Design review of the part built by this model. Coordinates are the model's own, in mm. A direction names the side the tool comes from. Coordinates: 2 decimals unless noted, no trailing zeros. Loops run counter-clockwise (first coordinate to the right, second up) from the corner with the lowest first, then second, coordinate; pieces in that order, holes last. Notation, with made-up numbers: M -6,86 L 27,86 A18 cw 27,91 Z; hole C 26.25,33.25 d7. An arc over 180 degrees is marked long. Answer as a JSON object with one key per item and string values. Group by question number.
1. Draft analysis for pull direction Z (two halves, no side actions). For faces 1 (the flat face through (10, 0, 0)), 2 (the flat face through (0, -10.922, 10)), 3 (the cylindrical face through (-0.123, 0.248, -12.303)), 4 (the flat face through (10, 0, 20.32)), state which applies: +Z half, -Z half, draft (parallel to the pull), parting line (faces both ways), or undercut.
2. Machinability: for faces 5 (the flat face through (-10, 0, 20.32)), 6 (the flat face through (8.763, -2, -7)), 7 (the flat face through (8.763, -2, 28)), which of the approach directions +Z, -Z, +X, -X, +Y, -Y give a long, thin tool a straight path to every point of the face, cutting with its end or side? Answer none if there is none.
3. Insertion check: pin 1 (3 mm diameter, centred on x = -5, z = -6, fed in from +Y); pin 2 (3 mm diameter, centred on x = 10, y = -3, fed in from -Z); pin 3 (3 mm diameter, centred on x = -10.5, y = 3, fed in from +Z); pin 4 (3 mm diameter, centred on y = 0, z = -10.414, fed in from -X). Each pin has a flat end and moves straight along its axis. Give the tip position at first contact, or say it passes through.
4. Consider section C-C (z = -2). State the section outline as (x, y) points.
5. Consider section A-A (y = 5.5). State the section outline as (x, z) points, then the cut area to 3 significant figures.
6. To check wall thickness, follow probe 1 along Z at (x, y) = (2.25, 0); probe 2 along X at (y, z) = (-6.35, -4.5); probe 3 along Y at (x, z) = (1.25, 1). State the ranges of each line that lie inside material, in increasing order.
7. Consider section D-D (x = 0). Count the separate pieces of the cut face and the enclosed holes in it, then the cut area to 3 significant figures.
8. Consider section B-B (x = -3.5). State the section outline as (y, z) points (3 decimals), then the cut area to 3 significant figures.
from build123d import *

# Parameters (mm, degrees)
SKETCH1_R               = 12.7
FINGERBODY_DEPTH        = 20.32
SKETCH2_W               = 17.526
SKETCH2_H               = 18.384757926
BOSS_EXTRUDE2_DEPTH     = 16.51
SKETCH4_R               = 1.905
CUT_EXTRUDE2_DEPTH      = 45.479200409
CUT_EXTRUDE3_DEPTH      = 45.479200409
FILLET2_R               = 2.54
CUT_EXTRUDE5_DEPTH      = 41.975955144
FILLET3_R               = 1.524
FILLET4_R               = 1.524
FILLET6_R               = 1.524
CUT_EXTRUDE6_DEPTH      = 41.460214887
CUT_EXTRUDE6_DEPTH_BACK = 41.460214887
SKETCH11_R              = 2.413


with BuildPart() as part:
    # Sketch1 → FingerBody (new body)
    with BuildSketch(Plane.XY):
        Circle(SKETCH1_R)
    extrude(amount=FINGERBODY_DEPTH)

    # Sketch2 → Boss-Extrude2 (add)
    with BuildSketch(Plane(origin=(0, 0, 0), x_dir=(-1, 0, 0), z_dir=(0, 0, -1))):
        Rectangle(SKETCH2_W, SKETCH2_H)
    boss_extrude2 = extrude(amount=BOSS_EXTRUDE2_DEPTH)

    # Mirror1: Boss-Extrude2 across plane
    add(boss_extrude2.mirror(Plane(origin=(0, 0, 10.16), x_dir=(1, 0, 0), z_dir=(0, 0, -1))))

    # Sketch4 → Cut-Extrude2 (cut, through all)
    with BuildSketch(Plane.ZY.offset(8.763)):
        with Locations(Location((30.734, 0, 0), (0, 0, 270))):
            Circle(SKETCH4_R)
    cut_extrude2 = extrude(amount=-CUT_EXTRUDE2_DEPTH, mode=Mode.SUBTRACT)

    # Mirror2: Cut-Extrude2 across plane
    add(cut_extrude2.mirror(Plane(origin=(0, 0, 10.16), x_dir=(1, 0, 0), z_dir=(0, 0, -1))), mode=Mode.SUBTRACT)

    # Sketch5 → Cut-Extrude3 (cut, through all)
    with BuildSketch(Plane(origin=(8.763, 0, 0), x_dir=(0, 0, -1), z_dir=(1, 0, 0))):
        Polygon((16.51, 1.572378963), (0.508, 9.192378963), (16.51, 9.192378963), align=None)
    cut_extrude3 = extrude(amount=-CUT_EXTRUDE3_DEPTH, mode=Mode.SUBTRACT)

    # Fillet2
    fillet2_edges = [part.edges().sort_by_distance(p)[0] for p in [
        (0, -9.192378963, -16.51),
        (8.763, -3.81, -16.51),
        (0, 1.572378963, -16.51),
        (-8.763, -3.81, -16.51),
    ]]
    fillet(fillet2_edges, radius=FILLET2_R)

    # Mirror6: Cut-Extrude3 across plane
    add(cut_extrude3.mirror(Plane(origin=(0, 0, 10.16), x_dir=(1, 0, 0), z_dir=(0, 0, -1))), mode=Mode.SUBTRACT)

    # Sketch8 → Cut-Extrude5 (cut, symmetric)
    with BuildSketch(Plane(origin=(0, 0, 0), x_dir=(-1, 0, 0), z_dir=(0, 0, -1))):
        with BuildLine():
            Line((6.480734218, 10.922), (-6.480734218, 10.922))
            ThreePointArc((-6.480734218, 10.922), (0, 12.7), (6.480734218, 10.922))
        make_face()
    cut_extrude5 = extrude(amount=CUT_EXTRUDE5_DEPTH, both=True, mode=Mode.SUBTRACT)

    # Mirror7: Cut-Extrude5 across plane
    add(cut_extrude5.mirror(Plane(origin=(0, 0, 0), x_dir=(0, 0, 1), z_dir=(0, -1, 0))), mode=Mode.SUBTRACT)

    # Fillet3
    fillet3_edges = [part.edges().sort_by_distance(p)[0] for p in [
        (6.480734218, 10.922, 10.16),
        (-6.480734218, 10.922, 10.16),
        (0, 10.922, 20.32),
        (0, 10.922, 0),
    ]]
    fillet(fillet3_edges, radius=FILLET3_R)

    # Fillet4
    fillet4_edges = [part.edges().sort_by_distance(p)[0] for p in [
        (6.480734218, -10.922, 10.16),
        (-6.480734218, -10.922, 10.16),
        (0, -10.922, 20.32),
        (0, -10.922, 0),
    ]]
    fillet(fillet4_edges, radius=FILLET4_R)

    # Fillet6
    fillet6_edges = [part.edges().sort_by_distance(p)[0] for p in [
        (-8.763, -3.81, 36.83),
        (0, -9.192378963, 36.83),
        (8.763, -3.81, 36.83),
        (0, 1.572378963, 36.83),
    ]]
    fillet(fillet6_edges, radius=FILLET6_R)

    # Sketch11 → Cut-Extrude6 (cut, two sides: drawn at the far end of the back side and taken through both)
    with BuildSketch(Plane.XY.offset(20.32).offset(-CUT_EXTRUDE6_DEPTH_BACK)):
        with Locations(Location((0, 6.35, 0), (0, 0, 270))):
            Circle(SKETCH11_R)
        with Locations(Location((0, -6.35, 0), (0, 0, 352.801199766))):
            Circle(SKETCH11_R)
    extrude(amount=CUT_EXTRUDE6_DEPTH + CUT_EXTRUDE6_DEPTH_BACK, mode=Mode.SUBTRACT)


solid = part.part
Findings below:
{
 "1": {"face 1": "-Z half", "face 2": "draft", "face 3": "undercut", "face 4": "+Z half"},
 "2": {"face 5": "+Z, -X, +Y, -Y", "face 6": "-Z, +X, +Y, -Y", "face 7": "+Z, +X, +Y, -Y"},
 "3": {"pin 1": "stops at y = 7.29", "pin 2": "stops at z = -15.1", "pin 3": "stops at z = 20.32", "pin 4": "passes through"},
 "4": {"outline": "M -8.76,-9.19 L 8.76,-9.19 L 8.76,8.48 L 1.13,8.48 A2.41 cw long -1.13,8.48 L -8.76,8.48 Z; hole C 0,-6.35 d4.83"},
 "5": {"outline": "M -11.45,0 L -8.76,0 L -8.76,-8.26 L -2.26,-8.26 L -2.26,28.58 L -8.76,28.58 L -8.76,20.32 L -11.45,20.32 Z; M 2.26,-8.26 L 8.76,-8.26 L 8.76,0 L 11.45,0 L 11.45,20.32 L 8.76,20.32 L 8.76,28.58 L 2.26,28.58 Z", "area": "588 mm^2"},
 "6": {"probe 1": "z = -16.51 to -12.32, -8.51 to 28.83, 32.64 to 36.83", "probe 2": "x = -8.76 to -2.41, 2.41 to 8.76", "probe 3": "y = -10.83 to -8.41, -4.29 to 4.29, 8.41 to 10.83"},
 "7": {"separate pieces": "3", "enclosed holes": "2", "area": "485 mm^2"},
 "8": {"outline": "M -10.922,1.524 A1.524 ccw -9.398,0 L -9.192,0 L -9.192,-13.97 A2.54 ccw -6.652,-16.51 L -0.031,-16.51 A2.54 ccw 2.262,-15.062 L 9.192,-0.508 L 9.192,0 L 9.398,0 A1.524 ccw 10.922,1.524 L 10.922,18.796 A1.524 ccw 9.398,20.32 L 9.192,20.32 L 9.192,20.828 L 1.986,35.961 A1.524 ccw 0.61,36.83 L -7.668,36.83 A1.524 ccw -9.192,35.306 L -9.192,20.32 L -9.398,20.32 A1.524 ccw -10.922,18.796 Z; hole C 0,-10.414 d3.81; hole C 0,30.734 d3.81", "area": "902 mm^2"}
}
